Geometry check sheet. Reference: drawing and pictorial views, mm from the part's lowest x, y, z. A direction names the side the tool comes from. Coordinates: 2 decimals unless noted, no trailing zeros. Write each loop counter-clockwise with the first axis right and the second up, starting at its lowest first coordinate (ties: lowest second). Pieces come first, ordered by that corner, then holes. Notation, with made-up numbers: (50.25, 37.25) -> (57.25, 37.25) arc R20 cw to (57.25, 72.25) -> close; hole circle Ø3 at (31.5, 31). An arc over 180 degrees is marked (long way). Use a Markdown table: item, result.
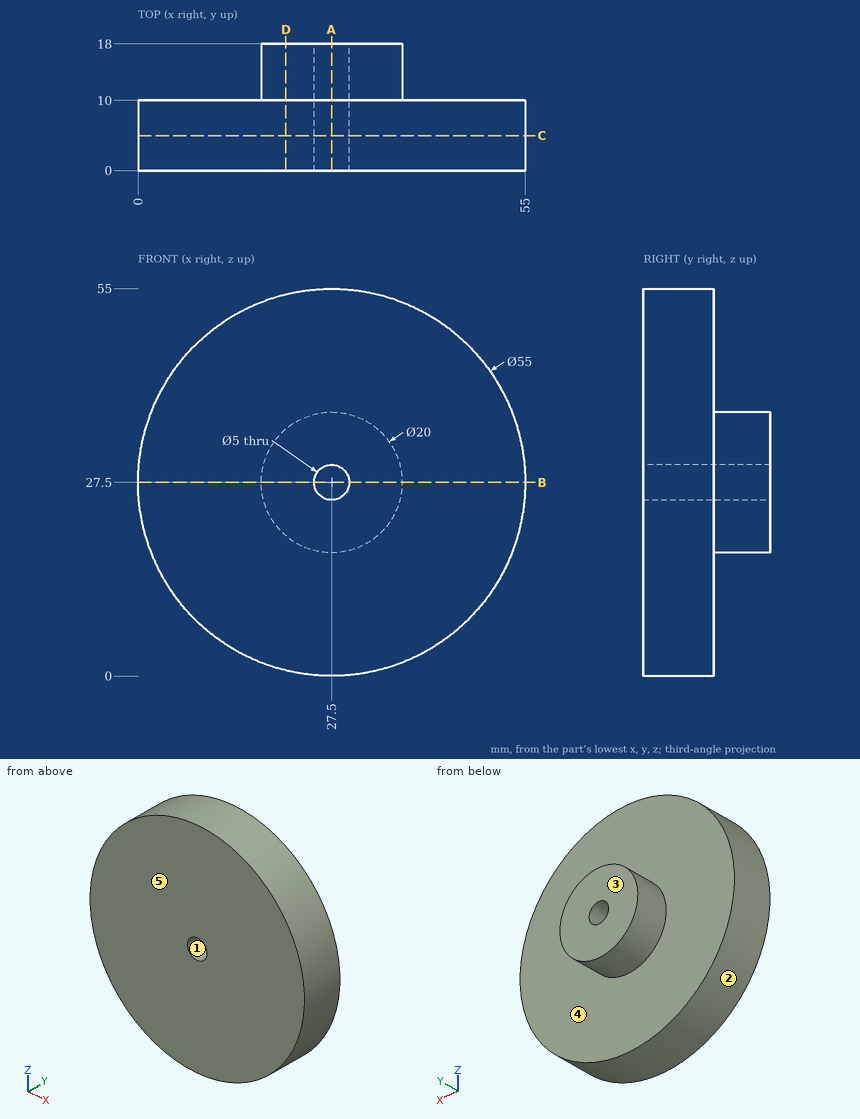
Item 1: Section check D-D on x = 21. Record the boundary of the cut face in (y, z), then the cut area to 3 significant figures.
Answer block:
| item | result |
|---|---|
| outline | (0, 0.78) -> (10, 0.78) -> (10, 19.9) -> (18, 19.9) -> (18, 35.1) -> (10, 35.1) -> (10, 54.22) -> (0, 54.22) -> close |
| area | 656 mm^2 |
Item 2: Thickness scan on L1, parallel to X at y = 13, z = 27.5; L2, parallel to X at y = 8, z = 27.5; L3, parallel to Y at x = 31, z = 52.5. Record the ranges inside material, lowest first. Write a range as [from, to].
Answer block:
| item | result |
|---|---|
| L1 | x = [17.5, 25], [30, 37.5] |
| L2 | x = [0, 25], [30, 55] |
| L3 | y = [0, 10] |
Item 3: Section check B-B on z = 27.5. Record the boundary of the cut face in (x, y).
Answer block:
| item | result |
|---|---|
| outline | (0, 0) -> (25, 0) -> (25, 18) -> (17.5, 18) -> (17.5, 10) -> (0, 10) -> close; (30, 0) -> (55, 0) -> (55, 10) -> (37.5, 10) -> (37.5, 18) -> (30, 18) -> close |
Item 4: Section check C-C on y = 5. Record the boundary of the cut face in (x, z).
Answer block:
| item | result |
|---|---|
| outline | circle Ø55 at (27.5, 27.5); hole circle Ø5 at (27.5, 27.5) |
Item 5: Tool access check on the marked faces 4 and 5. Record the directions out of +Z, -Z, +X, -X, +Y, -Y that give a thin tool (end or side, any length) a straight path to the whole face; none if there is none.
Answer block:
| item | result |
|---|---|
| face 4 | +Y |
| face 5 | +Z, -Z, +X, -X, -Y |
Item 6: Mould release check, pull along X, two halves, no side actions. Record for the marked faces 1, 2 and 3: +X half, -X half, draft (parallel to the pull), parting line (faces both ways), or undercut.
Answer block:
| item | result |
|---|---|
| face 1 | undercut |
| face 2 | parting line |
| face 3 | draft |
Item 7: Depth check by flat-ended pin: P1, Ø8, axis at x = 46, y = 6, coming from the +Z side; P2, Ø5, axis at y = 3, z = 7.5, coming from the -X side; P3, Ø3, axis at x = 38, z = 47.5, coming from the +Y side; P4, Ø2, axis at x = 25.5, z = 47.5, coming from the -Y side. Enter the tip coordinate at first touch or a pass-through.
Answer block:
| item | result |
|---|---|
| P1 | stops at z = 50.87 |
| P2 | stops at x = 6.29 |
| P3 | stops at y = 10 |
| P4 | stops at y = 0 |
Item 8: Section check A-A on x = 27.5. Record the boundary of the cut face in (y, z).
Answer block:
| item | result |
|---|---|
| outline | (0, 0) -> (10, 0) -> (10, 17.5) -> (18, 17.5) -> (18, 25) -> (0, 25) -> close; (0, 30) -> (18, 30) -> (18, 37.5) -> (10, 37.5) -> (10, 55) -> (0, 55) -> close |
